Build history of the part. All positions in model axes, mm. Give positions to 0.01 mm unless a question says otherwise; leave off trailing zeros. Loops run counter-clockwise (first coordinate to the right, second up) from the corner with the lowest first, then second, coordinate; pieces in that order, holes last. Notation, with made-up numbers: M 54,-20.5 L 89,-20.5 A24 ccw 89,-1.5 Z; hole C 34,55 d8. An arc over 180 degrees is marked long. Put each result on its own line as item: value.
```python
from build123d import *

# Parameters (mm, degrees)
SKETCH_532_W           = 518
SKETCH_532_H           = 297
EXTRUDE_604_DEPTH      = 155
SKETCH_5_3_R           = 38.5
CUT_EXTRUDE_11_DEPTH   = 123
SKETCH_1_R             = 15
CUT_EXTRUDE_1423_DEPTH = 30


with BuildPart() as part:
    # Sketch 532 → Extrude 604 (new body)
    with BuildSketch(Plane(origin=(0, 0, 0), x_dir=(1, 0, 0), z_dir=(0, 1, 0))):
        with Locations((184, -92)):
            Rectangle(SKETCH_532_W, SKETCH_532_H)
    extrude(amount=-EXTRUDE_604_DEPTH)

    # Матрица 5*3 → Ложемент для КМЕ-11 (cut)
    with BuildSketch(Plane(origin=(0, 0, 0), x_dir=(1, 0, 0), z_dir=(0, 1, 0))):
        with Locations(Location((0, 0, 0), (0, 0, 270))):
            Circle(SKETCH_5_3_R)
        with Locations(Location((92, 0, 0), (0, 0, 270))):
            Circle(SKETCH_5_3_R)
        with Locations(Location((184, 0, 0), (0, 0, 270))):
            Circle(SKETCH_5_3_R)
        with Locations(Location((276, 0, 0), (0, 0, 270))):
            Circle(SKETCH_5_3_R)
        with Locations(Location((368, 0, 0), (0, 0, 270))):
            Circle(SKETCH_5_3_R)
        with Locations(Location((0, -92, 0), (0, 0, 270))):
            Circle(SKETCH_5_3_R)
        with Locations(Location((92, -92, 0), (0, 0, 270))):
            Circle(SKETCH_5_3_R)
        with Locations(Location((184, -92, 0), (0, 0, 270))):
            Circle(SKETCH_5_3_R)
        with Locations(Location((276, -92, 0), (0, 0, 270))):
            Circle(SKETCH_5_3_R)
        with Locations(Location((368, -92, 0), (0, 0, 270))):
            Circle(SKETCH_5_3_R)
        with Locations(Location((0, -184, 0), (0, 0, 270))):
            Circle(SKETCH_5_3_R)
        with Locations(Location((92, -184, 0), (0, 0, 270))):
            Circle(SKETCH_5_3_R)
        with Locations(Location((184, -184, 0), (0, 0, 270))):
            Circle(SKETCH_5_3_R)
        with Locations(Location((276, -184, 0), (0, 0, 270))):
            Circle(SKETCH_5_3_R)
        with Locations(Location((368, -184, 0), (0, 0, 270))):
            Circle(SKETCH_5_3_R)
    extrude(amount=-CUT_EXTRUDE_11_DEPTH, mode=Mode.SUBTRACT)

    # Эскиз1 → Cut-Extrude 1423 (cut)
    with BuildSketch(Plane(origin=(0, 0, 0), x_dir=(1, 0, 0), z_dir=(0, 1, 0))):
        with Locations((27.223611076, -27.223611076)):
            Circle(SKETCH_1_R)
        with Locations((-27.223611076, 27.223611076)):
            Circle(SKETCH_1_R)
        with Locations((119.223611076, -27.223611076)):
            Circle(SKETCH_1_R)
        with Locations((64.776388924, 27.223611076)):
            Circle(SKETCH_1_R)
        with Locations((211.223611076, -27.223611076)):
            Circle(SKETCH_1_R)
        with Locations((156.776388924, 27.223611076)):
            Circle(SKETCH_1_R)
        with Locations((303.223611076, -27.223611076)):
            Circle(SKETCH_1_R)
        with Locations((248.776388924, 27.223611076)):
            Circle(SKETCH_1_R)
        with Locations((395.223611076, -27.223611076)):
            Circle(SKETCH_1_R)
        with Locations((340.776388924, 27.223611076)):
            Circle(SKETCH_1_R)
        with Locations((119.223611076, -119.223611076)):
            Circle(SKETCH_1_R)
        with Locations((64.776388924, -64.776388924)):
            Circle(SKETCH_1_R)
        with Locations((211.223611076, -119.223611076)):
            Circle(SKETCH_1_R)
        with Locations((156.776388924, -64.776388924)):
            Circle(SKETCH_1_R)
        with Locations((303.223611076, -119.223611076)):
            Circle(SKETCH_1_R)
        with Locations((248.776388924, -64.776388924)):
            Circle(SKETCH_1_R)
        with Locations((395.223611076, -119.223611076)):
            Circle(SKETCH_1_R)
        with Locations((340.776388924, -64.776388924)):
            Circle(SKETCH_1_R)
        with Locations((119.223611076, -211.223611076)):
            Circle(SKETCH_1_R)
        with Locations((64.776388924, -156.776388924)):
            Circle(SKETCH_1_R)
        with Locations((211.223611076, -211.223611076)):
            Circle(SKETCH_1_R)
        with Locations((156.776388924, -156.776388924)):
            Circle(SKETCH_1_R)
        with Locations((303.223611076, -211.223611076)):
            Circle(SKETCH_1_R)
        with Locations((248.776388924, -156.776388924)):
            Circle(SKETCH_1_R)
        with Locations((395.223611076, -211.223611076)):
            Circle(SKETCH_1_R)
        with Locations((340.776388924, -156.776388924)):
            Circle(SKETCH_1_R)
        with Locations((27.223611076, -119.223611076)):
            Circle(SKETCH_1_R)
        with Locations((-27.223611076, -64.776388924)):
            Circle(SKETCH_1_R)
        with Locations((27.223611076, -211.223611076)):
            Circle(SKETCH_1_R)
        with Locations((-27.223611076, -156.776388924)):
            Circle(SKETCH_1_R)
    extrude(amount=-CUT_EXTRUDE_1423_DEPTH, mode=Mode.SUBTRACT)


solid = part.part
```
Q1. Drop flat-ended pins along their axis: pin 1 Ø23 at (x, z) = (96.5, 181) entering from +Y; pin 2 Ø8 at (x, z) = (241.5, -30.5) entering from +Y; pin 3 Ø12 at (x, z) = (-15.5, 33.5) entering from +Y. Give the stop position or say it passes through.
Here are the results:
pin 1: y = -123
pin 2: y = -30
pin 3: y = 0
Q2. Slice it at C-C (x = 92). List the corners of the cut face in (y, z), and give its area (3 significant figures).
Here are the results:
outline: M -155,-56.5 L 0,-56.5 L 0,-38.5 L -123,-38.5 L -123,38.5 L 0,38.5 L 0,53.5 L -123,53.5 L -123,130.5 L 0,130.5 L 0,145.5 L -123,145.5 L -123,222.5 L 0,222.5 L 0,240.5 L -155,240.5 Z
area: 17,600 mm²
Q3. Probe line 1 (X direction, y = -27, z = 188.5); line 2 (X direction, y = -88, z = 74.5); line 3 (Z direction, x = 167, y = -84.5). List the from-to ranges inside material, lowest first. Write a range as from..to.
Here are the results:
line 1: -75..-38.24, 38.24..53.76, 130.24..145.76, 222.24..237.76, 314.24..329.76, 406.24..443
line 2: -75..-34.29, 34.29..57.71, 126.29..149.71, 218.29..241.71, 310.29..333.71, 402.29..443
line 3: -56.5..-34.54, 34.54..57.46, 126.54..149.46, 218.54..240.5
Q4. Slice it at A-A (y = -51.5). State how many separate pieces and enclosed holes the cut face has, and give its area (3 significant figures).
Here are the results:
separate pieces: 1
enclosed holes: 15
area: 84,000 mm²
Q5. Slice it at B-B (z = 0). List the corners of the cut face in (x, y).
Here are the results:
outline: M -75,-155 L 443,-155 L 443,0 L 406.5,0 L 406.5,-123 L 329.5,-123 L 329.5,0 L 314.5,0 L 314.5,-123 L 237.5,-123 L 237.5,0 L 222.5,0 L 222.5,-123 L 145.5,-123 L 145.5,0 L 130.5,0 L 130.5,-123 L 53.5,-123 L 53.5,0 L 38.5,0 L 38.5,-123 L -38.5,-123 L -38.5,0 L -75,0 Z
Q6. Mould opens along X. For faces 1 (the cylindrical face through (54.435, -14.79, 145.911)), 2 (the flat face through (152, -30, 152)), 3 (the flat face through (180, -76, 240.5)) say: pulls with the +X half, pulls with the -X half, needs draft (parallel to the pull), parting line crosses it, or undercut.
Here are the results:
face 1: undercut
face 2: undercut
face 3: needs draft
Q7. Slice it at D-D (x = 389). List the corners of the cut face in (y, z).
Here are the results:
outline: M -155,-56.5 L 0,-56.5 L 0,-32.27 L -123,-32.27 L -123,32.27 L -30,32.27 L -30,40.87 L 0,40.87 L 0,59.73 L -123,59.73 L -123,124.27 L -30,124.27 L -30,132.87 L 0,132.87 L 0,151.73 L -123,151.73 L -123,216.27 L -30,216.27 L -30,224.87 L 0,224.87 L 0,240.5 L -155,240.5 Z
